The figure shows three views and two pictorial views of one solid part (mm, origin at its lowest corner). Answer the questions. Coordinates: 2 decimals unless noted, no trailing zeros. Write each loop counter-clockwise with the first axis right and the second up, starting at its lowest first coordinate (ties: lowest second). Pieces come first, ordered by that corner, then holes. Notation, with made-up numbers: M -15.75,36.25 L 18.25,36.25 A29 cw 18.25,56.25 Z; hole C 44.5,54 d3. An arc over 180 degrees is marked long. Answer as CSV lines item,"result".
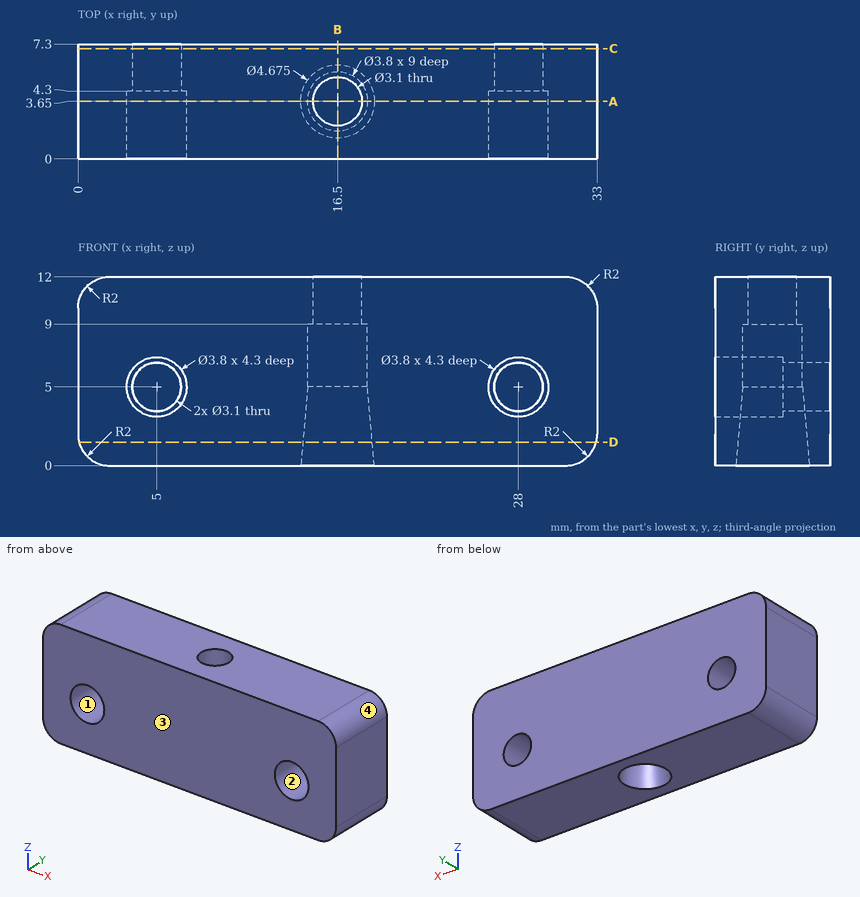
Q1. Find section D-D (z = 1.5). Give the vertices of the cut face in (x, y), and give its area (3 significant figures).
Output:
outline,"M 0.06,0 L 32.94,0 L 32.94,7.3 L 0.06,7.3 Z; hole C 16.5,3.65 d4.41"
area,"225 mm2"
Q2. Straight lines are drawn through the part: line 1 (X direction, y = 3.65, z = 6.2); line 2 (Y direction, x = 16.5, z = 10.9); line 3 (X direction, y = 3.5, z = 9.5). For each, find the intervals that lie inside material, in ascending order.
Output:
line 1,"0 to 3.53, 6.47 to 14.6, 18.4 to 26.53, 29.47 to 33"
line 2,"0 to 2.1, 5.2 to 7.3"
line 3,"0 to 14.96, 18.04 to 33"
Q3. Flat-ended cylindrical pins translate along their axes: pin 1 Ø2 at (x, y) = (29.5, 5) entering from -Z; pin 2 Ø1.1 at (x, y) = (15.5, 4) entering from -Z. Find the tip coordinate at first contact, or state that the pin passes through.
Output:
pin 1,"z = 0"
pin 2,"z = 9"
Q4. Find section A-A (y = 3.65). Give the vertices of the cut face in (x, z).
Output:
outline,"M 0,2 A2 ccw 2,0 L 14.16,0 L 14.6,5 L 14.6,9 L 14.95,9 L 14.95,12 L 2,12 A2 ccw 0,10 Z; M 18.05,9 L 18.4,9 L 18.4,5 L 18.84,0 L 31,0 A2 ccw 33,2 L 33,10 A2 ccw 31,12 L 18.05,12 Z; hole C 5,5 d3.8; hole C 28,5 d3.8"
Q5. Find section C-C (y = 7). Give the vertices of the cut face in (x, z), and give its area (3 significant figures).
Output:
outline,"M 0,2 A2 ccw 2,0 L 31,0 A2 ccw 33,2 L 33,10 A2 ccw 31,12 L 2,12 A2 ccw 0,10 Z; hole C 5,5 d3.1; hole C 28,5 d3.1"
area,"377 mm2"
Q6. The mould has two halves that part along X. Classify the marked faces 1, 2, 3 and 4: pulls with the +X half, pulls with the -X half, needs draft (parallel to the pull), parting line crosses it, or undercut.
Output:
face 1,"undercut"
face 2,"undercut"
face 3,"needs draft"
face 4,"pulls with the +X half"
Q7. Find section B-B (x = 16.5). Give the vertices of the cut face in (y, z), and give its area (3 significant figures).
Output:
outline,"M 0,0 L 1.31,0 L 1.75,5 L 1.75,9 L 2.1,9 L 2.1,12 L 0,12 Z; M 5.2,9 L 5.55,9 L 5.55,5 L 5.99,0 L 7.3,0 L 7.3,12 L 5.2,12 Z"
area,"41.9 mm2"
